Here's how the part is built. I have some questions about the finished solid (model axes, mm). Face numbers are marked on the shaded views. A direction names the side the tool comes from. Give positions to 0.01 mm unless a question says otherwise; leave off trailing zeros. Loops run counter-clockwise (first coordinate to the right, second up) from the corner with the lowest first, then second, coordinate; pieces in that order, holes last. Notation, with made-up numbers: (36, 11.25) - (85, 11.25) arc R31 cw to (85, 35.25) - close; hole circle Ø1 at (-24.5, -14). An arc over 180 degrees is marked (long way). Use a Markdown table: item, result.
from build123d import *

# Parameters (mm, degrees)
F0_W     = 50
F0_H     = 50
F1_DEPTH = 5
F2_W     = 5
F2_H     = 50
F3_DEPTH = 50
F4_W     = 50
F4_H     = 5
F5_DEPTH = 36.8
F6_W     = 3.2
F6_H     = 8.2
F7_DEPTH = 50


# Not quite as in the source:
# - a feature names something its author has since deleted; it is built from what else it names


with BuildPart() as f1:
    # F0 (on Top) → F1 (new body)
    with BuildSketch(Plane.XY):
        Rectangle(F0_W, F0_H)
    extrude(amount=F1_DEPTH)

    # F2 (on face) → F3 (join, through all)
    with BuildSketch(Plane(origin=(-25, 0, 0), x_dir=(0, -1, 0), z_dir=(-1, 0, 0))):
        with Locations((-22.5, -20)):
            Rectangle(F2_W, F2_H)
        with Locations((-14.3, -20)):
            Rectangle(F2_W, F2_H)
    extrude(amount=-F3_DEPTH)

    # F4 (on face) → F5 (join, through all)
    with BuildSketch(Plane.XZ.offset(-11.8)):
        with Locations((0, -5.7)):
            Rectangle(F4_W, F4_H)
    extrude(amount=F5_DEPTH)

    # F6 (on face) → F7 (join, through all)
    with BuildSketch(Plane(origin=(-25, 0, 0), x_dir=(0, -1, 0), z_dir=(-1, 0, 0))):
        with Locations((-18.4, -4.1)):
            Rectangle(F6_W, F6_H)
    extrude(amount=-F7_DEPTH)


solid = f1.part
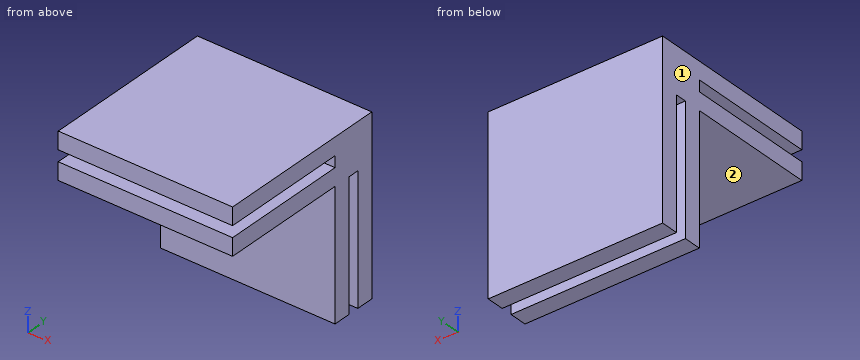
(1) If I drill on line 1 (Z direction, x = 7, y = 3.5); line 2 (Y direction, x = 6.5, z = -15); line 3 (Y direction, x = 22.5, z = -1.5), over which ranges is the centre line in solid material (lowest first)?
A:
| item | result |
|---|---|
| line 1 | -8.2 to -3.2, 0 to 5 |
| line 2 | 11.8 to 16.8, 20 to 25 |
| line 3 | 11.8 to 25 |
(2) Suppose I cut it at C-C on x = -1. Write out the boundary of the cut face in (y, z), plus the area to 3 significant figures.
A:
| item | result |
|---|---|
| outline | (-25, -8.2) - (11.8, -8.2) - (11.8, -45) - (16.8, -45) - (16.8, -8.2) - (20, -8.2) - (20, -45) - (25, -45) - (25, 5) - (-25, 5) - (-25, 0) - (11.8, 0) - (11.8, -3.2) - (-25, -3.2) - close |
| area | 910 mm2 |
(3) Will these pins go through, and if not, where does the flat tip stop? pin 1 (18.5 mm diameter, centred on x = 1.5, z = -18, fed in from -Y); pin 2 (5 mm diameter, centred on x = 12, z = -2.5, fed in from -Y); pin 3 (12 mm diameter, centred on x = 8.5, y = -18.5, fed in from -Z).
A:
| item | result |
|---|---|
| pin 1 | y = 11.8 |
| pin 2 | y = -25 |
| pin 3 | z = -8.2 |
(4) On a 3-axis mill with a long thin cutter (end or side, diameter ignored), from which of +Z, -Z, +X, -X, +Y, -Y can I reach the whole of each face in a straight line? I mean the marked faces 1 and 2. Say none if no direction works.
A:
| item | result |
|---|---|
| face 1 | +Z, -Z, -X, +Y, -Y |
| face 2 | -Z, +X, -X, -Y |
(5) Suppose I cut it at B-B on y = 7.5. Write out the boundary of the cut face in (x, z), plus the area to 3 significant figures.
A:
| item | result |
|---|---|
| outline | (-25, -8.2) - (25, -8.2) - (25, -3.2) - (-25, -3.2) - close; (-25, 0) - (25, 0) - (25, 5) - (-25, 5) - close |
| area | 500 mm2 |
(6) Suppose I cut it at A-A on z = -35. Write out the boundary of the cut face in (x, y).
A:
| item | result |
|---|---|
| outline | (-25, 11.8) - (25, 11.8) - (25, 16.8) - (-25, 16.8) - close; (-25, 20) - (25, 20) - (25, 25) - (-25, 25) - close |
